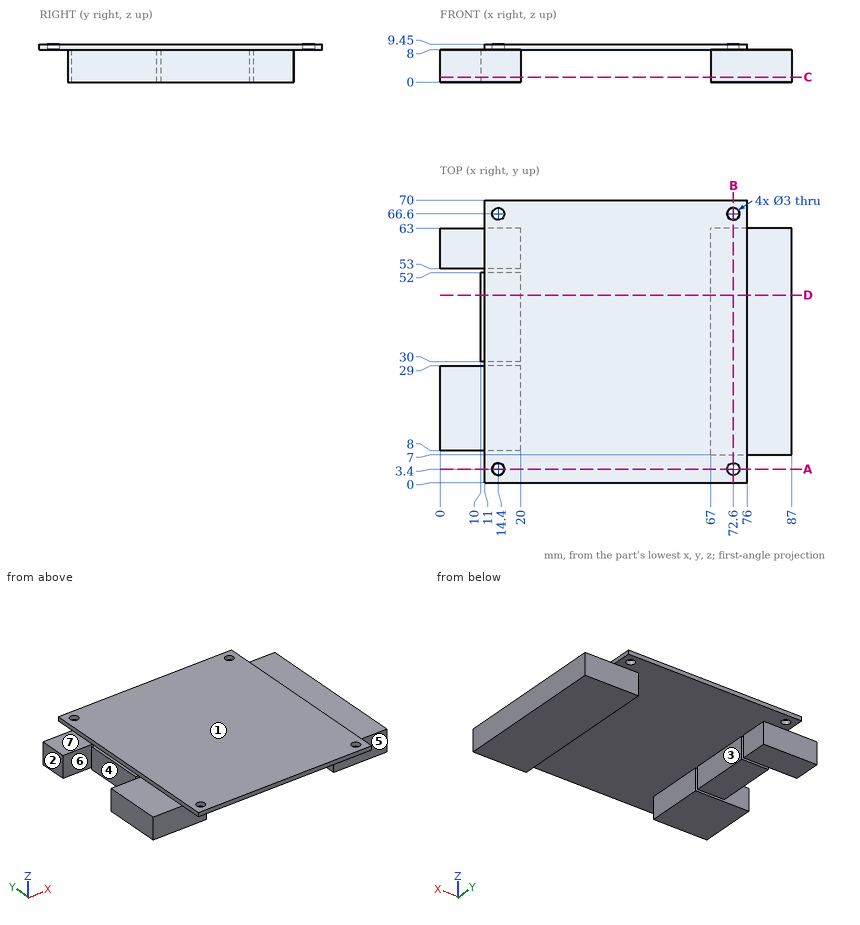
Drawing for the job (mm, zero at the part's lowest x, y, z). A direction names the side the tool comes from. Give positions to 0.01 mm unless a question says otherwise; leave off trailing zeros. Loops run counter-clockwise (first coordinate to the right, second up) from the corner with the lowest first, then second, coordinate; pieces in that order, holes last.
1) Band-saw the part on D-D on y = 46.5. List the corners of the cut face in (x, z).
Values follow:
outline: (10, 0) - (20, 0) - (20, 8) - (67, 8) - (67, 0) - (87, 0) - (87, 8) - (76, 8) - (76, 9.45) - (11, 9.45) - (11, 8) - (10, 8) - close
2) 3-axis set-ups, long thin cutter, end or side, ignore diameter. For the marked faces 4, 5, 6 and 7: which of +Z, -Z, +X, -X, +Y, -Y reach the whole face in a straight line?
Values follow:
face 4: +Z, -Z, -X
face 5: -Z, +X, -X, -Y
face 6: -Z, -X
face 7: +Z, -X, +Y, -Y
3) Band-saw the part on A-A on y = 3.4. List the corners of the cut face in (x, z).
Values follow:
outline: (11, 8) - (12.9, 8) - (12.9, 9.45) - (11, 9.45) - close; (15.9, 8) - (71.1, 8) - (71.1, 9.45) - (15.9, 9.45) - close; (74.1, 8) - (76, 8) - (76, 9.45) - (74.1, 9.45) - close
4) Probe line 1 along X through (y, z) = (66.6, 8.3); line 2 along Y through (x, z) = (72.6, 9.1); line 3 along X through (y, z) = (43.5, 2.25). List the from-to ranges inside material, lowest first.
Values follow:
line 1: x = 11 to 12.9, 15.9 to 71.1, 74.1 to 76
line 2: y = 0 to 1.9, 4.9 to 65.1, 68.1 to 70
line 3: x = 10 to 20, 67 to 87
5) Band-saw the part on C-C on z = 1.25. List the corners of the cut face in (x, y), then the cut area to 3 significant figures.
Values follow:
outline: (0, 8) - (20, 8) - (20, 29) - (0, 29) - close; (0, 53) - (20, 53) - (20, 63) - (0, 63) - close; (10, 30) - (20, 30) - (20, 52) - (10, 52) - close; (67, 7) - (87, 7) - (87, 63) - (67, 63) - close
area: 1,960 mm2
6) Drop flat-ended pins along their axis: P1, Ø1.2, axis at y = 31.5, z = 9, coming from the +X side; P2, Ø5, axis at x = 72.6, y = 66.6, coming from the -Z side; P3, Ø9, axis at x = 4.5, y = 15, coming from the +Z side. Give the stop position or say it passes through.
Values follow:
P1: stops at x = 76
P2: stops at z = 8
P3: stops at z = 8
7) Band-saw the part on B-B on x = 72.6. List the corners of the cut face in (y, z), then the cut area to 3 significant figures.
Values follow:
outline: (0, 8) - (1.9, 8) - (1.9, 9.45) - (0, 9.45) - close; (4.9, 8) - (7, 8) - (7, 0) - (63, 0) - (63, 8) - (65.1, 8) - (65.1, 9.45) - (4.9, 9.45) - close; (68.1, 8) - (70, 8) - (70, 9.45) - (68.1, 9.45) - close
area: 541 mm2
8) Two-plate mould, pull along X, no slides. Class the marked faces 1, 2 and 3: released by +X, released by -X, zero draft, split by the parting line, or undercut.
Values follow:
face 1: zero draft
face 2: released by -X
face 3: undercut
